Autodesk Inventor part; units mm, degrees
ref_plane "YZ Plane" through (0, 0, 0) normal (1, 0, 0) x (0, 1, 0)
ref_plane "XZ Plane" through (0, 0, 0) normal (0, 1, 0) x (-1, 0, 0)
ref_plane "XY Plane" through (0, 0, 0) normal (0, 0, 1) x (1, 0, 0)
sketch "Sketch1" plane through (0, 0, 0) normal (0, 0, 1) x (1, 0, 0)
  arc A0 (670.9948, -199.4141) -> (0, 0) centre (254.9219, -370.8299) ccw
  arc A1 (657.7848, -239.4141) -> (30, 0) centre (229.3296, -420.1103) ccw
  arc A2 (657.7848, -239.4141) -> (670.9948, -199.4141) centre (0, 0) ccw
  line L0 (0, 0) -> (30, 0)
  line L1 (657.7848, -239.4141) -> (0, 0)
  line L2 (-143.7228, 0) -> (862.3369, 0)
  point P0 (0, 0)
  dimension "d1" = 30
  dimension "d2" = 40
  dimension "d4" = 20
  dimension "d5" = 465
  dimension "d6" = 450
  dimension "d22" = 700
extrude "Extrusion1" add sketch "Sketch1" along normal blind 4 contours A2 A1 L2 A0 | L2 A1 L0 A0
sketch "Sketch2" plane through (0, 0, 4) normal (0, 0, 1) x (1, 0, 0)
  arc A0 (670.9948, -199.4141) -> (0, 0) centre (254.9219, -370.8299) ccw
  arc A1 (87.1309, 22.5434) -> (74.166, 50.9844) centre (0, 0) ccw
  line L0 (74.166, 50.9844) -> (0, 0)
  line L1 (0, 0) -> (87.1309, 22.5434)
  line L2 (0, 0) -> (30, 0)
  point P0 (78.8927, 43.3122)
  point P1 (0, 0)
  point P2 (0, 0)
  dimension "d9" = 90
  dimension "d16" = 20
extrude "Extrusion2" add sketch "Sketch2" against normal blind 4
sketch "Sketch4" plane through (0, 0, 4) normal (0, 0, 1) x (1, 0, 0)
  line L0 (86.0304, 22.2587) -> (87.1309, 22.5434)
  line L1 (74.166, 50.9844) -> (0, 0)
  line L2 (87.1309, 22.5434) -> (0, 0)
  line L3 (0, 0) -> (30, 0)
  arc A0 (86.0304, 22.2587) -> (30, 0) centre (229.3296, -420.1103) ccw
  line L4 (30, 0) -> (86.0304, 22.2587)
  point P0 (86.0304, 22.2587)
extrude "Extrusion4" cut sketch "Sketch4" against normal blind 10 contours A0 L3 L2
sketch "Sketch5" plane through (0, 0, 4) normal (0, 0, 1) x (1, 0, 0)
  line L0 (0, 0) -> (20.6017, 14.1623)
  line L1 (74.166, 50.9844) -> (0, 0)
  line L2 (0, 0) -> (87.1309, 22.5434)
  line L3 (24.203, 6.2621) -> (0, 0)
  arc A0 (24.203, 6.2621) -> (20.6017, 14.1623) centre (0, 0) ccw
  point P0 (24.203, 6.2621)
  dimension "d21" = 25
extrude "Extrusion5" cut sketch "Sketch5" against normal blind 10
sketch "Sketch6" plane through (0, 0, 4) normal (0, 0, 1) x (1, 0, 0)
  circle A0 centre (37.1637, 14.7938) radius 1.5
  circle A1 centre (71.4659, 35.9531) radius 1.5
  circle A2 centre (76.6234, 22.9969) radius 1.5
  line L0 (37.1637, 14.7938) -> (0, 0)
  line L1 (0, 0) -> (71.4659, 35.9531)
  line L2 (76.6234, 22.9969) -> (0, 0)
  line L3 (24.203, 6.2621) -> (87.1309, 22.5434)
  line L4 (74.166, 50.9844) -> (20.6017, 14.1623)
  line L5 (0, 0) -> (261.3927, 67.6302)
  line L6 (0, 0) -> (264.574, 53.8573)
  circle A3 centre (260.1726, 72.1818) radius 1.5
  circle A4 centre (264.574, 53.8573) radius 1.5
  circle A5 centre (281.2279, 70.1567) radius 1.5
  circle A6 centre (285.6292, 51.8321) radius 1.5
  line L7 (281.2279, 70.1567) -> (285.6292, 51.8321)
  line L8 (285.6292, 51.8321) -> (264.574, 53.8573)
  line L9 (264.574, 53.8573) -> (260.1726, 72.1818)
  line L10 (260.1726, 72.1818) -> (281.2279, 70.1567)
  line L11 (260.1726, 72.1818) -> (0, 0)
  dimension "d23" = 3
  dimension "d24" = 3
  dimension "d25" = 3
  dimension "d26" = 7.2
  dimension "d27" = 2.2
  dimension "d28" = 7.8
  dimension "d29" = 40
  dimension "d30" = 80
  dimension "d31" = 80
  dimension "d34" = 3
  dimension "d35" = 270
  dimension "d36" = 270
  dimension "d37" = 3
  dimension "d38" = 3
  dimension "d39" = 20
  dimension "d40" = 109
  dimension "d41" = 3
  dimension "d42" = 3
  dimension "d43" = 1
  dimension "d44" = 270
extrude "Extrusion6" cut sketch "Sketch6" against normal blind 10 contours A0 | A2 | A1 | A4 L9 L6 | L6 L8 A4 | L11 L9 A3 | A3 L10 L11 | L9 A4 L8 | L9 L10 A3 | L8 L7 A6 | A6 L7 L8 | L10 L7 A5 | A5 L7 L10
sketch "Sketch7" plane through (0, 0, 4) normal (0, 0, 1) x (1, 0, 0)
  line L0 (20.6017, 14.1623) -> (74.166, 50.9844)
  arc A0 (78.8927, 43.3122) -> (74.166, 50.9844) centre (0, 0) ccw
  line L1 (20.6017, 14.1623) -> (74.166, 50.9844)
  line L2 (74.166, 50.9844) -> (82.5313, 50.9844)
  arc A1 (21.2689, 13.139) -> (20.6017, 14.1623) centre (0, 0) ccw
  line L3 (21.2689, 13.139) -> (82.5313, 50.9844)
  line L4 (21.2689, 13.139) -> (0, 0)
  line L5 (0, 0) -> (20.6017, 14.1623)
  point P0 (76.568, 47.3005)
  dimension "d45" = 2.8
extrude "Extrusion7" cut sketch "Sketch7" against normal blind 10 contours L0 A0 L3 A1
sketch "Sketch8" plane through (0, 0, 4) normal (0, 0, 1) x (1, 0, 0)
  line L0 (87.1309, 22.5434) -> (24.203, 6.2621)
  line L1 (24.203, 6.2621) -> (87.1309, 22.5434)
  arc A0 (24.48, 5.0723) -> (24.203, 6.2621) centre (0, 0) ccw
  arc A1 (88.1281, 18.2602) -> (87.1309, 22.5434) centre (0, 0) ccw
  line L2 (88.1281, 18.2602) -> (24.48, 5.0723)
  line L3 (24.48, 5.0723) -> (0, 0)
  arc A2 (24.203, 6.2621) -> (21.2689, 13.139) centre (0, 0) ccw
  line L4 (0, 0) -> (24.203, 6.2621)
  arc A3 (78.8927, 43.3122) -> (76.568, 47.3005) centre (0, 0) ccw
  dimension "d48" = 2.8
extrude "Extrusion8" add sketch "Sketch8" against normal blind 4 contours A1 L2 A0 L0
properties part number "spoke"
Work out the finished part from the listing and answer in its coordinate system (mm). Round coordinates to 2 decimals unless told otherwise and drop trailing zeros. Write each loop counter-clockwise with the first axis right and the second up, starting at its lowest first coordinate (ties: lowest second). Pieces come first, ordered by that corner, then holes.
1) A flat-ended cylindrical pin translates along its axis: P1, Ø1.5, axis at y = -74, z = 3, coming from the -X side. Find the tip coordinate at first contact, or state that the pin passes through.
2) A cutting plane is placed at A-A on z = 1.55. Determine the outline of the cut face in (x, y).
3) A cutting plane is placed at C-C on x = 333.5. Determine the outline of the cut face in (y, z), and give its area (3 significant figures).
4) A cutting plane is placed at B-B on y = -1.5. Determine the outline of the cut face in (x, z).
5) Consider probe 1 along Y at (x, z) = (77, 0.6); probe 2 along X at (y, z) = (-38.5, 1.8); probe 3 along Y at (x, z) = (476, 0.75). Determine where each line is inside the solid, lowest interval first.
6) Determine the mould class of faces 1 (the face through (417, 15, 4)), 2 (the face through (664.783, -219.233, 1.972)), 3 (the face through (56.75, 11.76, 2.03)) for opening direction X: pulls with the +X half, pulls with the -X half, needs draft (parallel to the pull), parting line crosses it, or undercut.
Entries:
1. P1: stops at x = 539.03
2. outline: (21.27, 13.14) arc R25 cw to (24.2, 6.26) arc R25.02 cw to (24.48, 5.07) - (88.13, 18.26) arc R90.02 ccw to (87.13, 22.54) arc R90 ccw to (87.11, 22.61) arc R465 cw to (657.78, -239.41) arc R700.04 ccw to (670.99, -199.41) arc R450 ccw to (78.89, 43.31) arc R90 ccw to (76.57, 47.3) - close; hole circle Ø3 at (37.16, 14.79); hole circle Ø3 at (71.47, 35.95); hole circle Ø3 at (76.62, 23); hole circle Ø3 at (260.17, 72.18); hole circle Ø3 at (264.57, 53.86); hole circle Ø3 at (281.23, 70.16); hole circle Ø3 at (285.63, 51.83)
3. outline: (33.07, 0) - (72.26, 0) - (72.26, 4) - (33.07, 4) - close
3. area: 157 mm2
4. outline: (431.79, 0) - (512.01, 0) - (512.01, 4) - (431.79, 4) - close
5. probe 1: y = 15.95 to 21.54, 24.45 to 46.59
5. probe 2: x = 495.03 to 558.33
5. probe 3: y = -25.93 to 21.12
6. face 1: needs draft
6. face 2: pulls with the +X half
6. face 3: undercut
